```python
from build123d import *

# Parameters (mm, degrees)
PAD_DEPTH       = 10
SKETCH001_R     = 8
POCKET_DEPTH    = 5
SKETCH003_R     = 6
POCKET001_DEPTH = 5
POCKET002_DEPTH = 10
FILLET_R        = 1


with BuildPart() as part:
    # Sketch → Pad (new body)
    with BuildSketch(Plane.XY):
        with BuildLine():
            Line((40, 0), (-40, 0))
            Line((-40, 0), (-40, 15))
            Line((-9.661357, 48.698171), (-40, 15))
            ThreePointArc((9.661357, 48.698171), (0, 53), (-9.661357, 48.698171))
            Line((9.661357, 48.698171), (40, 15))
            Line((40, 0), (40, 15))
        make_face()
    extrude(amount=PAD_DEPTH)

    # Sketch001 (on Face7 of Pad) → Pocket (cut)
    with BuildSketch(Plane(origin=(0, 0, 0), x_dir=(1, 0, 0), z_dir=(0, 0, -1))):
        with Locations((0, -40)):
            Circle(SKETCH001_R)
    extrude(amount=-POCKET_DEPTH, mode=Mode.SUBTRACT)

    # Sketch003 (on Face10 of Pocket) → Pocket001 (cut)
    with BuildSketch(Plane(origin=(0, 0, 5), x_dir=(1, 0, 0), z_dir=(0, 0, -1))):
        with Locations((0, -40)):
            Circle(SKETCH003_R)
    extrude(amount=-POCKET001_DEPTH, mode=Mode.SUBTRACT)

    # Sketch002 (on Face4 of Pocket001) → Pocket002 (cut)
    with BuildSketch(Plane(origin=(0, 0, 0), x_dir=(1, 0, 0), z_dir=(0, 0, -1))):
        Polygon((-40, -15), (-40, 0), (-25, 0), (-25, -10), (-30, -10), (-30, -5), (-35, -5), (-35, -15), align=None)
        Polygon((40, -15), (40, 0), (25, 0), (25, -10), (30, -10), (30, -5), (35, -5), (35, -15), align=None)
    extrude(amount=-POCKET002_DEPTH, mode=Mode.SUBTRACT)

    # Fillet
    fillet_edges = [part.edges().sort_by_distance(p)[0] for p in [
        (37.5, 15, 10),
        (24.830678, 31.849086, 0),
    ]]
    fillet(fillet_edges, radius=FILLET_R)


solid = part.part
```
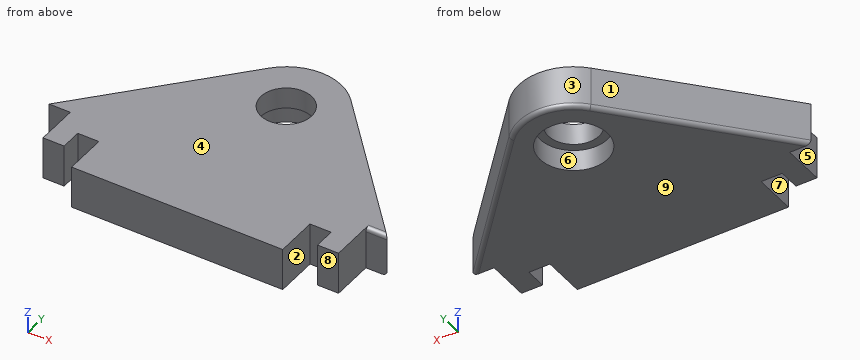
The model under review builds one solid part; all positions refer to its coordinate system, in mm. Face numbers are marked on the shaded views. A direction names the side the tool comes from. Give positions to 0.01 mm unless a question says otherwise; leave off trailing zeros. Write each loop counter-clockwise with the first axis right and the second up, starting at its lowest first coordinate (ties: lowest second). Pieces come first, ordered by that corner, then holes.
(1) Consider section B-B, the plane z = 4. Give the boundary of the cut face in (x, y), and give its area (3 significant figures).
(2) For P1, Ø7, axis at x = 0, y = 40, coming from the +Z side; P2, Ø4, axis at x = 18.5, z = 6, coming from the +Y side; P3, Ø5.5, axis at y = 8.5, z = 3, coming from the +X side; P4, Ø1.5, axis at y = 6.5, z = 4, coming from the -X side, all flat-tipped, find the tip position at first contact; note any pin that passes through.
(3) To check wall thickness, follow L1, parallel to Y at x = 0, z = 7.95; L2, parallel to Y at x = 0.5, z = 3.5; L3, parallel to X at y = 40, z = 3.9. State the ranges of each line that lie inside material, in increasing order.
(4) The part is to be moulded in two halves that separate along X. For the marked faces 1, 2, 3 and 4, say which applies: released by +X, released by -X, zero draft, split by the parting line, or undercut.
(5) Tool access review of the marked faces 5, 6, 7, 8 and 9: name each direction out of +Z, -Z, +X, -X, +Y, -Y from which nothing blocks a thin tool from reaching the whole face with its end or side.
(6) Consider section A-A, the plane x = 0. Give the boundary of the cut face in (y, z), and give its area (3 significant figures).
Returned:
1. outline: (-40, 15) - (-35, 15) - (-35, 5) - (-30, 5) - (-30, 10) - (-25, 10) - (-25, 0) - (25, 0) - (25, 10) - (30, 10) - (30, 5) - (35, 5) - (35, 15) - (40, 15) - (9.66, 48.7) arc R13 ccw to (-9.66, 48.7) - close; hole circle Ø16 at (0, 40)
1. area: 2,430 mm2
2. P1: passes through
2. P2: stops at y = 41.1
2. P3: stops at x = 35
2. P4: stops at x = -35
3. L1: y = 0 to 34, 46 to 53
3. L2: y = 0 to 32.02, 47.98 to 52.99
3. L3: x = -17.49 to -8, 8 to 17.49
4. face 1: released by -X
4. face 2: undercut
4. face 3: split by the parting line
4. face 4: zero draft
5. face 5: +Z, -Z, -X, -Y
5. face 6: -Z
5. face 7: +Z, -Z, -Y
5. face 8: +Z, -Z, +X, -Y
5. face 9: -Z, +X, -X, +Y, -Y
6. outline: (0, 0) - (32, 0) - (32, 5) - (34, 5) - (34, 10) - (0, 10) - close; (46, 5) - (48, 5) - (48, 0) - (52, 0) arc R1 ccw to (53, 1) - (53, 10) - (46, 10) - close
6. area: 390 mm2
